Geometry: final body of the model. Coordinates: model frame, mm. A direction names the side the tool comes from. Coordinates: 2 decimals unless noted, no trailing zeros. Order: outer loops, then holes, each group sorted by start corner. A loop starts at its lowest first (then second) coordinate and runs counter-clockwise, first axis right, second up. Notation, with made-up numbers: (84, -26) - (109, -26) arc R17 cw to (109, -21) - close; hole circle Ø8 at (11, 53.25). An arc over 180 degrees is marked (long way). Use one line per item in the form item = value. Start each with the question number.
```python
from build123d import *

# Parameters (mm, degrees)
SKETCH_1_W      = 40
SKETCH_1_H      = 25
EXTRUDE_1_DEPTH = 15
SKETCH_2_W      = 9.169537909
SKETCH_2_H      = 25
EXTRUDE_2_DEPTH = 10
OTHER_1_DEPTH   = 25
SKETCH_6_R      = 3.5
EXTRUDE_3_DEPTH = 5
EXTRUDE_START   = 5
SKETCH_7_R      = 3.5
EXTRUDE_4_DEPTH = 5


# Read off the part's stored shape, not the designer's step: 边界1
with BuildPart() as part:
    # 草图1 → 凸台-拉伸1 (new body)
    with BuildSketch(Plane(origin=(0, 0, 0), x_dir=(1, 0, 0), z_dir=(0, 1, 0))):
        with Locations((20, -12.5)):
            Rectangle(SKETCH_1_W, SKETCH_1_H)
    extrude(amount=EXTRUDE_1_DEPTH)

    # 草图2 → 凸台-拉伸2 (add)
    with BuildSketch(Plane(origin=(0, 15, 0), x_dir=(1, 0, 0), z_dir=(0, 1, 0))):
        with Locations((4.584768955, -12.5)):
            Rectangle(SKETCH_2_W, SKETCH_2_H)
    extrude(amount=EXTRUDE_2_DEPTH)

    # 边界1 outline → 边界1 (add)
    with BuildSketch(Plane.XY):
        Polygon((9.169537909, 15), (40, 15), (9.169537909, 25), align=None)
    extrude(amount=OTHER_1_DEPTH)

    # 草图6 → 凸台-拉伸3 (add)
    with BuildSketch(Plane(origin=(0, 0, 0), x_dir=(-1, 0, 0), z_dir=(0, 0, -1))):
        with Locations(Location((-20, 8, 0), (0, 0, 180))):
            Circle(SKETCH_6_R)
    extrude(amount=EXTRUDE_3_DEPTH)

    # 草图7 → 凸台-拉伸4 (add)
    with BuildSketch(Plane.XY.offset(25).offset(EXTRUDE_START)):
        with Locations((20, 8)):
            Circle(SKETCH_7_R)
    extrude(amount=-EXTRUDE_4_DEPTH)


solid = part.part
```
(1) Cut plane B-B on z = 8. Return the cut outline in (x, y), plus the area to 3 significant figures.
(2) Cut plane A-A on y = 8. Return the cut outline in (x, z).
(3) Set-up query: faces 1 (the cylindrical face through (21.615, 4.895, 27.535)), 2 (the cylindrical face through (23.233, 9.341, -2.465)), 3 (the flat face through (20, 0, 12)). Return all of +Z, -Z, +X, -X, +Y, -Y with unobstructed straight access to the full face (end or side cutting, diameter ignored); none if empty.
(4) Material intervals for L1, parallel to Z at x = 12, y = 5; L2, parallel to Y at x = 28, z = 23; L3, parallel to Y at x = 38, z = 14.5, sorted ascending. Write a range as from..to.
(5) Contact query for flat-ended pins moving along their axis: pin 1 Ø3 at (x, y) = (4.5, 5.5) entering from +Z; pin 2 Ø2 at (x, z) = (15, 0.5) entering from +Y. Output: stop coordinate, or through.
(6) Cut plane D-D on x = 3. Return the cut outline in (y, z), plus the area to 3 significant figures.
(7) Cut plane C-C on x = 20. Return the cut outline in (y, z).
Check sheet entries:
q1.outline = (0, 0) - (40, 0) - (40, 15) - (9.17, 25) - (0, 25) - close
q1.area = 846 mm^2
q2.outline = (0, 0) - (16.5, 0) - (16.5, -5) - (23.5, -5) - (23.5, 0) - (40, 0) - (40, 25) - (23.5, 25) - (23.5, 30) - (16.5, 30) - (16.5, 25) - (0, 25) - close
q3.face_1 = +Z
q3.face_2 = -Z
q3.face_3 = +Z, -Z, +X, -X, -Y
q4.L1 = 0..25
q4.L2 = 0..18.89
q4.L3 = 0..15.65
q5.pin_1 = 25
q5.pin_2 = 23.43
q6.outline = (0, 0) - (25, 0) - (25, 25) - (0, 25) - close
q6.area = 625 mm^2
q7.outline = (0, 0) - (4.5, 0) - (4.5, -5) - (11.5, -5) - (11.5, 0) - (21.49, 0) - (21.49, 25) - (11.5, 25) - (11.5, 30) - (4.5, 30) - (4.5, 25) - (0, 25) - close
